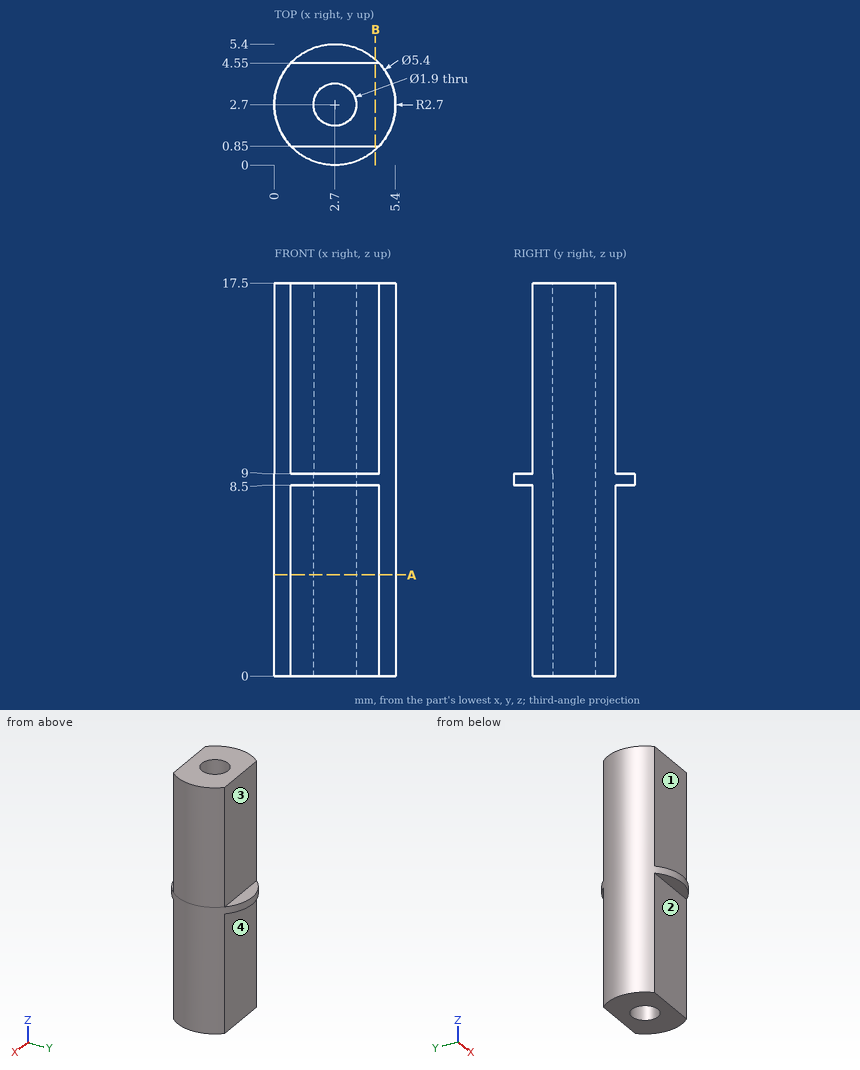
Geometry: see drawing. Coordinates: mm, zero at the bounding-box minimum. A direction names the side the tool comes from. Give positions to 0.01 mm unless a question says otherwise; leave off trailing zeros. Order: outer loops, then holes, each group sorted by start corner. A loop starts at its lowest first (then second) coordinate and runs counter-clockwise, first axis right, second up.
Q1. Section B-B on x = 4.5. Output: boundary loops of the cut face in (y, z), and give its area (3 significant figures).
Checked values:
outline: (0.69, 8.5) - (0.85, 8.5) - (0.85, 0) - (4.55, 0) - (4.55, 8.5) - (4.71, 8.5) - (4.71, 9) - (4.55, 9) - (4.55, 17.5) - (0.85, 17.5) - (0.85, 9) - (0.69, 9) - close
area: 64.9 mm2
Q2. Section A-A on z = 4.5. Output: boundary loops of the cut face in (x, y), and give its area (3 significant figures).
Checked values:
outline: (0.73, 0.85) - (4.67, 0.85) arc R2.7 ccw to (4.67, 4.55) - (0.73, 4.55) arc R2.7 ccw to start; hole circle Ø1.9 at (2.7, 2.7)
area: 15.4 mm2
Q3. Set-up query: the marked faces 1, 2, 3 and 4. Return all of +Z, -Z, +X, -X, +Y, -Y with unobstructed straight access to the full face (end or side cutting, diameter ignored); none if empty.
Checked values:
face 1: +Z, +X, -X, -Y
face 2: -Z, +X, -X, -Y
face 3: +Z, +X, -X, +Y
face 4: -Z, +X, -X, +Y
Q4. Ray query, probe 1 along Y at (x, z) = (2.7, 6.5); probe 2 along Y at (x, z) = (1.2, 16.75); probe 3 along Z at (x, y) = (3.05, 0.35). Return the intervals inside material, ascending.
Checked values:
probe 1: y = 0.85 to 1.75, 3.65 to 4.55
probe 2: y = 0.85 to 4.55
probe 3: z = 8.5 to 9
Q5. Contact query for flat-ended pins moving along their axis: pin 1 Ø2 at (x, z) = (3, 5.5) entering from +Y; pin 2 Ø1.5 at (y, z) = (1, 8.5) entering from +X; pin 3 Ø0.7 at (x, y) = (2.5, 5) entering from +Z. Output: stop coordinate, or through.
Checked values:
pin 1: stops at y = 4.55
pin 2: stops at x = 5.23
pin 3: stops at z = 9
